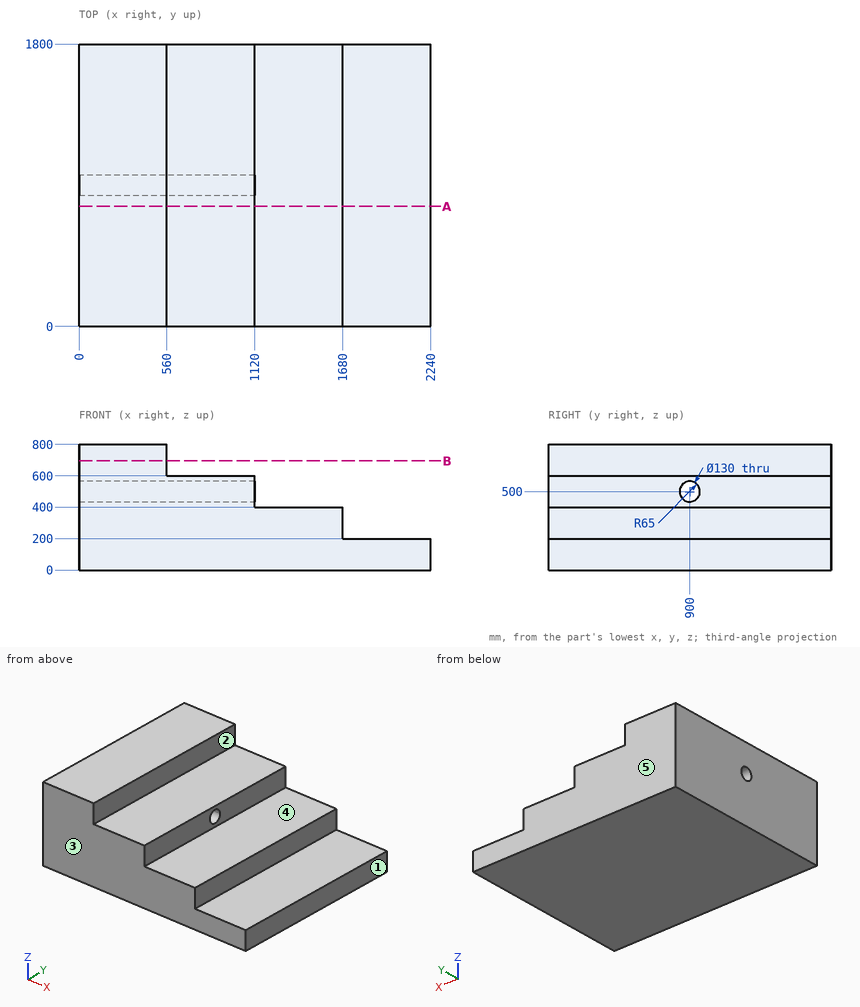
Print and shaded views of the part. All mm, measured from the part's lowest x, y and z. A direction names the side the tool comes from. Round coordinates to 2 decimals unless told otherwise and drop trailing zeros. Write each loop counter-clockwise with the first axis right and the second up, starting at its lowest first coordinate (ties: lowest second). Pieces come first, ordered by that corner, then holes. Notation, with made-up numbers: (-20, -39) - (-16, -39) arc R20 ccw to (-16, -28) - close; hole circle Ø5 at (77.5, -8.75). An arc over 180 degrees is marked (long way). Use CSV: the item, a comma, the result in double quotes. Start each with the question number.
Item 1: Band-saw the part on A-A (y = 766). Write the cut outline in (x, z).
Item 2: Two-plate mould, pull along Y, no slides. Class the marked faces 3, 4 and 5: released by +Y, released by -Y, zero draft, split by the parting line, or undercut.
Item 3: Band-saw the part on B-B (z = 696). Write the cut outline in (x, y).
Item 4: Pin check, flat tips, straight feed: P1, Ø1, axis at y = 786, z = 556.5, coming from the +X side; P2, Ø10, axis at x = 859, y = 760, coming from the +Z side; P3, Ø3, axis at y = 311.5, z = 189, coming from the -X side. Stop position of each tip, or through.
Item 5: Drill centre lines: L1, parallel to Z at x = 714.5, y = 900; L2, parallel to Y at x = 389, z = 500; L3, parallel to X at y = 81, z = 533. Where is each one in solid material? Low to high. Write a range as [from, to].
Item 6: Tool access for the marked faces 1 and 2: list every direction of +Z, -Z, +X, -X, +Y, -Y with a clear straight run to the whole face (end or side of a thin tool).
Checked values:
1,outline,"(0, 0) - (2240, 0) - (2240, 200) - (1680, 200) - (1680, 400) - (1120, 400) - (1120, 600) - (560, 600) - (560, 800) - (0, 800) - close"
2,face 3,"released by -Y"
2,face 4,"zero draft"
2,face 5,"released by +Y"
3,outline,"(0, 0) - (560, 0) - (560, 1800) - (0, 1800) - close"
4,P1,"stops at x = 1120"
4,P2,"stops at z = 600"
4,P3,"stops at x = 0"
5,L1,"z = [0, 435], [565, 600]"
5,L2,"y = [0, 835], [965, 1800]"
5,L3,"x = [0, 1120]"
6,face 1,"+Z, -Z, +X, +Y, -Y"
6,face 2,"+Z, +X, +Y, -Y"
